Geometry check sheet. Reference: the model listing, model coordinates, mm. A direction names the side the tool comes from. Round coordinates to 2 decimals unless told otherwise and drop trailing zeros. Write each loop counter-clockwise with the first axis right and the second up, starting at its lowest first coordinate (ties: lowest second). Pieces come first, ordered by that corner, then holes. Notation, with made-up numbers: (-17, 11) - (21, 11) arc R20 ccw to (21, 40) - close; hole circle Ø2 at (60.25, 44.5). An arc over 180 degrees is marked (long way). Return JSON: item names as keys, results as strings.
```python
from build123d import *

# Parameters (mm, degrees)
SKETCH1_W            = 698.5
SKETCH1_H            = 84.582
BOSS_EXTRUDE1_DEPTH  = 34.925
SKETCH2_W            = 81.407
SKETCH2_H            = 31.75
CUT_EXTRUDE1_DEPTH   = 699.5
SKETCH3_W            = 698.5
SKETCH3_H            = 3.175
BOSS_EXTRUDE2_DEPTH  = 50.8
M2_CLEARANCE_HOLE1_D = 2.54
M5_CLEARANCE_HOLE1_D = 5.334
CHAMFER1_SIZE        = 3.175
FILLET1_R            = 0.762
FILLET2_R            = 3.937
SKETCH8_W            = 848.789904452
SKETCH8_H            = 432.95839962
CUT_EXTRUDE2_DEPTH   = 85.582


with BuildPart() as part:
    # Sketch1 → Boss-Extrude1 (new body)
    with BuildSketch(Plane(origin=(0, 57.816398039, 0), x_dir=(1, 0, 0), z_dir=(0, 1, 0))):
        with Locations((253.148031467, -103.269491579)):
            Rectangle(SKETCH1_W, SKETCH1_H)
    extrude(amount=-BOSS_EXTRUDE1_DEPTH)

    # Sketch2 → Cut-Extrude1 (cut, through all)
    with BuildSketch(Plane(origin=(602.398031467, 0, 0), x_dir=(0, 0, -1), z_dir=(1, 0, 0))):
        with Locations((-101.681991579, 41.941398039)):
            Rectangle(SKETCH2_W, SKETCH2_H)
    extrude(amount=-CUT_EXTRUDE1_DEPTH, mode=Mode.SUBTRACT)

    # Sketch3 → Boss-Extrude2 (add)
    with BuildSketch(Plane(origin=(0, 26.066398039, 0), x_dir=(-1, 0, 0), z_dir=(0, 1, 0))):
        with Locations((-253.148031467, 62.565991579)):
            Rectangle(SKETCH3_W, SKETCH3_H)
    extrude(amount=BOSS_EXTRUDE2_DEPTH)

    # M2 Clearance Hole1 (through all)
    with Locations(Plane(origin=(0, 26.066398039, 0), x_dir=(1, 0, 0), z_dir=(0, 1, 0))):
        with Locations((-96.101968533, -136.543491579), (-96.101968533, -69.995491579)):
            Hole(M2_CLEARANCE_HOLE1_D / 2)

    # M5 Clearance Hole1 (through all)
    with Locations(Plane(origin=(0, 0, 60.978491579), x_dir=(-1, 0, 0), z_dir=(0, 0, -1))):
        with Locations((-469.048031467, 64.928398039), (-481.748031467, 64.928398039), (-469.048031467, 39.528398039), (-481.748031467, 39.528398039), (-456.348031467, 39.528398039), (-443.648031467, 39.528398039), (-430.948031467, 39.528398039), (-418.248031467, 39.528398039), (-405.548031467, 39.528398039), (-392.848031467, 39.528398039), (-380.148031467, 39.528398039), (-367.448031467, 39.528398039), (-354.748031467, 39.528398039), (-342.048031467, 39.528398039), (-329.348031467, 39.528398039), (-316.648031467, 39.528398039), (-303.948031467, 39.528398039), (-291.248031467, 39.528398039), (-278.548031467, 39.528398039), (-265.848031467, 39.528398039), (-253.148031467, 39.528398039), (-240.448031467, 39.528398039), (-227.748031467, 39.528398039), (-215.048031467, 39.528398039), (-202.348031467, 39.528398039), (-189.648031467, 39.528398039), (-176.948031467, 39.528398039), (-164.248031467, 39.528398039), (-151.548031467, 39.528398039), (-138.848031467, 39.528398039), (-126.148031467, 39.528398039), (-113.448031467, 39.528398039), (-100.748031467, 39.528398039), (-88.048031467, 39.528398039), (-75.348031467, 39.528398039), (-62.648031467, 39.528398039), (-49.948031467, 39.528398039), (-37.248031467, 39.528398039), (-24.548031467, 39.528398039), (-11.848031467, 39.528398039), (0.851968533, 39.528398039), (13.551968533, 39.528398039), (26.251968533, 39.528398039), (38.951968533, 39.528398039), (51.651968533, 39.528398039), (64.351968533, 39.528398039), (77.051968533, 39.528398039), (89.751968533, 39.528398039), (-456.348031467, 64.928398039), (-443.648031467, 64.928398039), (-430.948031467, 64.928398039), (-418.248031467, 64.928398039), (-405.548031467, 64.928398039), (-392.848031467, 64.928398039), (-380.148031467, 64.928398039), (-367.448031467, 64.928398039), (-354.748031467, 64.928398039), (-342.048031467, 64.928398039), (-329.348031467, 64.928398039), (-316.648031467, 64.928398039), (-303.948031467, 64.928398039), (-291.248031467, 64.928398039), (-278.548031467, 64.928398039), (-265.848031467, 64.928398039), (-253.148031467, 64.928398039), (-240.448031467, 64.928398039), (-227.748031467, 64.928398039), (-215.048031467, 64.928398039), (-202.348031467, 64.928398039), (-189.648031467, 64.928398039), (-176.948031467, 64.928398039), (-164.248031467, 64.928398039), (-151.548031467, 64.928398039), (-138.848031467, 64.928398039), (-126.148031467, 64.928398039), (-113.448031467, 64.928398039), (-100.748031467, 64.928398039), (-88.048031467, 64.928398039), (-75.348031467, 64.928398039), (-62.648031467, 64.928398039), (-49.948031467, 64.928398039), (-37.248031467, 64.928398039), (-24.548031467, 64.928398039), (-11.848031467, 64.928398039), (0.851968533, 64.928398039), (13.551968533, 64.928398039), (26.251968533, 64.928398039), (38.951968533, 64.928398039), (51.651968533, 64.928398039), (64.351968533, 64.928398039), (77.051968533, 64.928398039), (89.751968533, 64.928398039), (-494.448031467, 64.928398039), (-494.448031467, 39.528398039), (-507.148031467, 64.928398039), (-507.148031467, 39.528398039), (-519.848031467, 64.928398039), (-519.848031467, 39.528398039), (-532.548031467, 64.928398039), (-532.548031467, 39.528398039), (-545.248031467, 64.928398039), (-545.248031467, 39.528398039), (-557.948031467, 64.928398039), (-557.948031467, 39.528398039), (-570.648031467, 64.928398039), (-570.648031467, 39.528398039), (-583.348031467, 64.928398039), (-583.348031467, 39.528398039), (-596.048031467, 64.928398039), (-596.048031467, 39.528398039)):
            Hole(M5_CLEARANCE_HOLE1_D / 2)

    # Chamfer1
    chamfer1_edges = [part.edges().sort_by_distance(p)[0] for p in [
        (-96.101968533, 57.816398039, 143.972991579),
        (-96.101968533, 76.866398039, 62.565991579),
        (602.398031467, 76.866398039, 62.565991579),
        (602.398031467, 57.816398039, 143.972991579),
    ]]
    chamfer(chamfer1_edges, length=CHAMFER1_SIZE)

    # Fillet1
    fillet1_edges = [part.edges().sort_by_distance(p)[0] for p in [
        (253.148031467, 26.066398039, 142.385491579),
        (253.148031467, 26.066398039, 64.153491579),
    ]]
    fillet(fillet1_edges, radius=FILLET1_R)

    # Fillet2
    fillet2_edges = [part.edges().sort_by_distance(p)[0] for p in [
        (253.148031467, 22.891398039, 60.978491579),
        (253.148031467, 22.891398039, 145.560491579),
    ]]
    fillet(fillet2_edges, radius=FILLET2_R)

    # Sketch8 → Cut-Extrude2 (cut, through all)
    with BuildSketch(Plane(origin=(0, 0, 60.978491579), x_dir=(-1, 0, 0), z_dir=(0, 0, -1))):
        with Locations((-480.692983693, 24.593327381)):
            Rectangle(SKETCH8_W, SKETCH8_H)
    extrude(amount=-CUT_EXTRUDE2_DEPTH, mode=Mode.SUBTRACT)


solid = part.part
```
(1) Material ranges on line 1 along Z through (x, y) = (36, 47); line 2 along Y through (x, z) = (-11, 107); line 3 along X through (y, z) = (26, 136.5), recorded low to high. Write a range as [from, to].
Response values:
{"line 1": "z = [60.98, 64.15], [142.39, 145.56]", "line 2": "y = [22.89, 26.07]", "line 3": "x = [-94.83, 56.3]"}
(2) Section check C-C, the plane z = 79. Enter the section's corners in (x, y).
Response values:
{"outline": "(-96.1, 22.89) - (56.3, 22.89) - (56.3, 26.07) - (-96.1, 26.07) - close"}
(3) Gauge pin test, flat ends, axial feed: pin 1 (3 mm diameter, centred on x = -79, y = 65, fed in from +Z); pin 2 (3 mm diameter, centred on x = -14, z = 110, fed in from +Y). Record the tip position at first contact, or that the pin passes through.
Response values:
{"pin 1": "stops at z = 64.15", "pin 2": "stops at y = 26.07"}
(4) Section check A-A, the plane y = 51. Enter the section's corners in (x, z).
Response values:
{"outline": "(-96.1, 60.98) - (56.3, 60.98) - (56.3, 64.15) - (-96.1, 64.15) - close; (-96.1, 142.39) - (56.3, 142.39) - (56.3, 145.56) - (-96.1, 145.56) - close"}
(5) Release check for a two-part mould opening along X. For faces 1 (the face through (-74.5, 40.3, 144)), 2 (the face through (-94.537, 56.207, 143.995)), 3 (the face through (-21, 22.891, 103)), 4 (the face through (-1.199, 67.573, 62.588)) record: pulls with the +X half, pulls with the -X half, needs draft (parallel to the pull), parting line crosses it, or undercut.
Response values:
{"face 1": "undercut", "face 2": "pulls with the -X half", "face 3": "needs draft", "face 4": "undercut"}
(6) Access from +Z, -Z, +X, -X, +Y, -Y to the whole of each face (thin tool, end or side, straight path). Record for faces 5 (the face through (-18.835, 24.075, 62.101)), 6 (the face through (-19, 26.066, 104)).
Response values:
{"face 5": "-Z, +X, -X, -Y", "face 6": "+X, -X, +Y"}
(7) Section check B-B, the plane x = 5. Enter the section's corners in (y, z).
Response values:
{"outline": "(22.89, 64.92) arc R3.94 ccw to (26.83, 60.98) - (76.87, 60.98) - (76.87, 64.15) - (26.83, 64.15) arc R0.76 cw to (26.07, 64.92) - (26.07, 141.62) arc R0.76 cw to (26.83, 142.39) - (57.82, 142.39) - (57.82, 145.56) - (26.83, 145.56) arc R3.94 ccw to (22.89, 141.62) - close"}
